from build123d import *

# Parameters (mm, degrees)
F3_DEPTH = 39.624
F4_R     = 4.445
F5_DEPTH = 41.3102415224


with BuildPart() as f1:
    # F0 (on Front) → F1 (revolve)
    with BuildSketch(Plane.XZ):
        Polygon((17.4939688295, 0), (0, 0), (0, -2.54), (17.7669053052, -2.54), (46.9515744454, 3.8053627059), (46.9515744454, 38.7692414224), (44.4115744454, 38.7692414224), (44.4115744454, 5.8524552733), align=None)
    revolve(axis=Axis((0, 0, 19.3846207112), (0, 0, 1)))

    # F2 (on face) → F3 (join)
    with BuildSketch(Plane.XY.offset(38.7692414224)):
        with BuildLine():
            ThreePointArc((-7.5948700673, -46.333230964), (-0.3094269601, -54.5652893703), (7.62, -46.9515744454))
            ThreePointArc((7.62, -46.9515744454), (7.6137149248, -46.6421474854), (7.5948700673, -46.333230964))
            ThreePointArc((7.5948700673, -46.333230964), (0, -46.9515744454), (-7.5948700673, -46.333230964))
        make_face()
        with BuildLine():
            ThreePointArc((7.62, 46.9515744454), (-0.3094269601, 54.5652893703), (-7.5948700673, 46.333230964))
            ThreePointArc((-7.5948700673, 46.333230964), (0, 46.9515744454), (7.5948700673, 46.333230964))
            ThreePointArc((7.5948700673, 46.333230964), (7.6137149248, 46.6421474854), (7.62, 46.9515744454))
        make_face()
        with BuildLine():
            ThreePointArc((-46.333230964, 7.5948700673), (-54.5715744454, 0), (-46.333230964, -7.5948700673))
            ThreePointArc((-46.333230964, -7.5948700673), (-46.9515744454, 0), (-46.333230964, 7.5948700673))
        make_face()
        with BuildLine():
            ThreePointArc((-6.9655246042, -43.8619357953), (0, -44.4115744454), (6.9655246042, -43.8619357953))
            ThreePointArc((6.9655246042, -43.8619357953), (0, -39.3315744454), (-6.9655246042, -43.8619357953))
        make_face()
        with BuildLine():
            ThreePointArc((43.8619357953, 6.9655246042), (39.3315744454, 0), (43.8619357953, -6.9655246042))
            ThreePointArc((43.8619357953, -6.9655246042), (44.2739515495, -3.4935882577), (44.4115744454, 0))
            ThreePointArc((44.4115744454, 0), (44.2739515495, 3.4935882577), (43.8619357953, 6.9655246042))
        make_face()
        with BuildLine():
            ThreePointArc((-6.9655246042, 43.8619357953), (0, 39.3315744454), (6.9655246042, 43.8619357953))
            ThreePointArc((6.9655246042, 43.8619357953), (0, 44.4115744454), (-6.9655246042, 43.8619357953))
        make_face()
        with BuildLine():
            ThreePointArc((-43.8619357953, 6.9655246042), (-44.4115744454, 0), (-43.8619357953, -6.9655246042))
            ThreePointArc((-43.8619357953, -6.9655246042), (-40.5637952338, -4.1545970614), (-39.3315744454, 0))
            ThreePointArc((-39.3315744454, 0), (-40.5637952338, 4.1545970614), (-43.8619357953, 6.9655246042))
        make_face()
        with BuildLine():
            ThreePointArc((-7.5948700673, -46.333230964), (0, -46.9515744454), (7.5948700673, -46.333230964))
            ThreePointArc((7.5948700673, -46.333230964), (7.3843143351, -45.0710687156), (6.9655246042, -43.8619357953))
            ThreePointArc((6.9655246042, -43.8619357953), (0, -44.4115744454), (-6.9655246042, -43.8619357953))
            ThreePointArc((-6.9655246042, -43.8619357953), (-7.3843143351, -45.0710687156), (-7.5948700673, -46.333230964))
        make_face()
        with BuildLine():
            ThreePointArc((43.8619357953, -6.9655246042), (45.0710687156, -7.3843143351), (46.333230964, -7.5948700673))
            ThreePointArc((46.333230964, -7.5948700673), (46.7967332504, -3.81), (46.9515744454, 0))
            ThreePointArc((46.9515744454, 0), (46.7967332504, 3.81), (46.333230964, 7.5948700673))
            ThreePointArc((46.333230964, 7.5948700673), (45.0710687156, 7.3843143351), (43.8619357953, 6.9655246042))
            ThreePointArc((43.8619357953, 6.9655246042), (44.2739515495, 3.4935882577), (44.4115744454, 0))
            ThreePointArc((44.4115744454, 0), (44.2739515495, -3.4935882577), (43.8619357953, -6.9655246042))
        make_face()
        with BuildLine():
            ThreePointArc((7.5948700673, 46.333230964), (0, 46.9515744454), (-7.5948700673, 46.333230964))
            ThreePointArc((-7.5948700673, 46.333230964), (-7.3843143351, 45.0710687156), (-6.9655246042, 43.8619357953))
            ThreePointArc((-6.9655246042, 43.8619357953), (0, 44.4115744454), (6.9655246042, 43.8619357953))
            ThreePointArc((6.9655246042, 43.8619357953), (7.3843143351, 45.0710687156), (7.5948700673, 46.333230964))
        make_face()
        with BuildLine():
            ThreePointArc((-46.333230964, 7.5948700673), (-46.9515744454, 0), (-46.333230964, -7.5948700673))
            ThreePointArc((-46.333230964, -7.5948700673), (-45.0710687156, -7.3843143351), (-43.8619357953, -6.9655246042))
            ThreePointArc((-43.8619357953, -6.9655246042), (-44.4115744454, 0), (-43.8619357953, 6.9655246042))
            ThreePointArc((-43.8619357953, 6.9655246042), (-45.0710687156, 7.3843143351), (-46.333230964, 7.5948700673))
        make_face()
        with BuildLine():
            ThreePointArc((46.9515744454, 0), (46.7967332504, -3.81), (46.333230964, -7.5948700673))
            ThreePointArc((46.333230964, -7.5948700673), (52.116485997, -5.6025073551), (54.5715744454, 0))
            ThreePointArc((54.5715744454, 0), (52.116485997, 5.6025073551), (46.333230964, 7.5948700673))
            ThreePointArc((46.333230964, 7.5948700673), (46.7967332504, 3.81), (46.9515744454, 0))
        make_face()
    extrude(amount=-F3_DEPTH)

    # F4 (on face) → F5 (cut, through all)
    with BuildSketch(Plane.XY.offset(38.7692414224)):
        with Locations((-46.9515744454, 0)):
            Circle(F4_R)
        with Locations((0, 46.9515744454)):
            Circle(F4_R)
        with Locations((46.9515744454, 0)):
            Circle(F4_R)
        with Locations((0, -46.9515744454)):
            Circle(F4_R)
    extrude(amount=-F5_DEPTH, mode=Mode.SUBTRACT)


solid = f1.part
Work out the finished part from the listing and answer in its coordinate system (mm). A direction names the side the tool comes from. Give positions to 0.01 mm unless a question says otherwise; leave off trailing zeros. Loops run counter-clockwise (first coordinate to the right, second up) from the corner with the lowest first, then second, coordinate; pieces in that order, holes last. Notation, with made-up numbers: (74, 51) -> (98, 51) arc R29 cw to (98, 74) -> close; hole circle Ø6 at (65, 57.25). An arc over 180 degrees is marked (long way). Use a Markdown table: item, result. Add a question column.
1. Determine the mould class of faces 1 (the flat face through (40, 0, 38.769)), 2 (the cylindrical face through (-0.123, 39.333, 21.997)), 3 (the cylindrical face through (-33.488, -32.909, 21.532)) for opening direction X: released by +X, released by -X, zero draft, split by the parting line, or undercut.
2. Section A-A on z = 8 is taken. Determine the outline of the cut face in (x, y) (3 decimals).
3. Flat-ended cylindrical pins translate along their axes: pin 1 Ø1.5 at (x, z) = (37, 4) entering from -Y; pin 2 Ø17 at (x, y) = (-1, -47.5) entering from -Z; pin 3 Ø12 at (x, y) = (6.5, 6.5) entering from +Z; pin 4 Ø5.5 at (x, y) = (0, -46.95) entering from -Z. Find the tip coordinate at first contact, or state that the pin passes through.
4. Section B-B on x = 0 is taken. Determine the outline of the cut face in (y, z).
5. Section C-C on x = -48 is taken. Determine the outline of the cut face in (y, z).
6. Find the intervals of material crossed by probe 1 along Y at (x, z) = (0, 10); probe 2 along Y at (x, z) = (-40.5, 8.5); probe 3 along Y at (x, z) = (1, 35.5), in increasing order.
7. For faces 4 (the cylindrical face through (-32.909, 33.488, 21.532)), 5 (the flat face through (3.3, -50.2, -0.855)), 6 (the flat face through (-43.7, -3.3, -0.855)), 7 (the cylindrical face through (0.123, -39.333, 21.997)), determine the directions among +Z, -Z, +X, -X, +Y, -Y from which every point of the face is accessible in a straight line to the end or side of a thin tool.
Results below:
| question | item | result |
|---|---|---|
| 1 | face 1 | zero draft |
| 1 | face 2 | undercut |
| 1 | face 3 | released by -X |
| 2 | outline | (-46.333, -7.595) arc R46.952 ccw to (-7.595, -46.333) arc R7.62 ccw (long way) to (7.595, -46.333) arc R46.952 ccw to (46.333, -7.595) arc R7.62 ccw (long way) to (46.333, 7.595) arc R46.952 ccw to (7.595, 46.333) arc R7.62 ccw (long way) to (-7.595, 46.333) arc R46.952 ccw to (-46.333, 7.595) arc R7.62 ccw (long way) to start; hole circle Ø8.89 at (-46.952, 0); hole (-43.862, -6.966) arc R44.412 ccw to (-6.966, -43.862) arc R7.62 cw to (6.966, -43.862) arc R44.412 ccw to (43.862, -6.966) arc R7.62 cw to (43.862, 6.966) arc R44.412 ccw to (6.966, 43.862) arc R7.62 cw to (-6.966, 43.862) arc R44.412 ccw to (-43.862, 6.966) arc R7.62 cw to start; hole circle Ø8.89 at (0, -46.952); hole circle Ø8.89 at (0, 46.952); hole circle Ø8.89 at (46.952, 0) |
| 3 | pin 1 | stops at y = -29.84 |
| 3 | pin 2 | stops at z = -0.85 |
| 3 | pin 3 | stops at z = 0 |
| 3 | pin 4 | passes through |
| 4 | outline | (-54.57, -0.85) -> (-51.4, -0.85) -> (-51.4, 38.77) -> (-54.57, 38.77) -> close; (-42.51, -0.85) -> (-39.33, -0.85) -> (-39.33, 2.15) -> (-17.77, -2.54) -> (17.77, -2.54) -> (39.33, 2.15) -> (39.33, -0.85) -> (42.51, -0.85) -> (42.51, 38.77) -> (39.33, 38.77) -> (39.33, 4.75) -> (17.49, 0) -> (-17.49, 0) -> (-39.33, 4.75) -> (-39.33, 38.77) -> (-42.51, 38.77) -> close; (51.4, -0.85) -> (54.57, -0.85) -> (54.57, 38.77) -> (51.4, 38.77) -> close |
| 5 | outline | (-7.55, -0.85) -> (-4.32, -0.85) -> (-4.32, 38.77) -> (-7.55, 38.77) -> close; (4.32, -0.85) -> (7.55, -0.85) -> (7.55, 38.77) -> (4.32, 38.77) -> close |
| 6 | probe 1 | y = -54.57 to -51.4, -42.51 to -39.33, 39.33 to 42.51, 51.4 to 54.57 |
| 6 | probe 2 | y = -23.75 to -18.22, -4.05 to 4.05, 18.22 to 23.75 |
| 6 | probe 3 | y = -54.51 to -51.28, -42.62 to -39.4, 39.4 to 42.62, 51.28 to 54.51 |
| 7 | face 4 | +Z, -Z, -X, +Y |
| 7 | face 5 | -Z, +X, -X, -Y |
| 7 | face 6 | -Z, -X, +Y, -Y |
| 7 | face 7 | +Z |
